Verification items for the finished model (mm, model axes). A direction names the side the tool comes from. Coordinates: 2 decimals unless noted, no trailing zeros. Write each loop counter-clockwise with the first axis right and the second up, starting at its lowest first coordinate (ties: lowest second). Pieces come first, ordered by that corner, then holes. Notation, with made-up numbers: (9.25, 45.5) -> (31.25, 45.5) arc R17 cw to (31.25, 50.5) -> close; hole circle Ø11 at (55.5, 83). An arc over 180 degrees is marked (long way). Answer in a Markdown table with one row per item.
Autodesk Inventor part; units mm, degrees
ref_plane "Work Plane1" through (0, 12, 0) normal (0, 1, 0) x (1, 0, 0)
ref_plane "YZ Plane" through (0, 0, 0) normal (1, 0, 0) x (0, 1, 0)
ref_plane "XZ Plane" through (0, 0, 0) normal (0, 1, 0) x (-1, 0, 0)
sketch "Sketch1" plane through (0, 0, 0) normal (0, 1, 0) x (-1, 0, 0)
  line L0 (0, 8.6603) -> (7.5, 4.3301)
  line L1 (7.5, 4.3301) -> (7.5, -4.3301)
  line L2 (7.5, -4.3301) -> (0, -8.6603)
  line L3 (0, -8.6603) -> (-7.5, -4.3301)
  line L4 (-7.5, -4.3301) -> (-7.5, 4.3301)
  line L5 (-7.5, 4.3301) -> (0, 8.6603)
  point P0 (0, 0)
  point P1 (0, 0)
  dimension "d0" = 7.5
extrude "Extrusion1" add sketch "Sketch1" along normal blind 6
ref_plane "Work Plane1" through (0, 12, 0) normal (0, 1, 0) x (1, 0, 0)
sketch "Sketch3" plane through (0, 12, 0) normal (0, 1, 0) x (1, 0, 0)
  circle A0 centre (0, 0) radius 0.75
  dimension "d4" = 1.5
loft "Loft1" add profiles "Sketch3" section 1 edges at (-3.75, 6, 6.4952) (3.75, 6, 6.4952) (7.5, 6, 0) (3.75, 6, -6.4952) (-3.75, 6, -6.4952) (-7.5, 6, 0)
sketch "Sketch4" plane through (0, 0, 0) normal (0, -1, 0) x (1, 0, 0)
  circle A0 centre (0, 0) radius 5
  dimension "d9" = 10
extrude "Extrusion2" cut sketch "Sketch4" against normal blind 6
thread "Thread1"
sketch "Sketch5" plane through (0, 6, 0) normal (0, -1, 0) x (1, 0, 0)
  circle A0 centre (0, 0) radius 5
  circle A1 centre (0, 0) radius 1.5875
  dimension "d14" = 3.175
sketch "Sketch6" plane through (0, 12, 0) normal (0, 1, 0) x (1, 0, 0)
  arc A0 (-0.6495, 0.375) -> (-0.6495, -0.375) centre (0, 0) ccw
  circle A1 centre (0, 0) radius 0.175
  dimension "d15" = 0.35
extrude "Extrusion3" cut sketch "Sketch6" against normal blind 7.75
extrude "Extrusion4" cut sketch "Sketch5" against normal blind 3.9 contours A1
chamfer "Chamfer1" distance 1.4 angle 45 1 edges at (-0.175, 9.9, 0)
properties part number "Nozzle"
1. Tool access check on faces 5 (the cylindrical face through (-0.34, 7.92, -1.55)), 6 (the flat face through (7.5, 3, 0)). Record the directions out of +Z, -Z, +X, -X, +Y, -Y that give a thin tool (end or side, any length) a straight path to the whole face; none if there is none.
Geometry says:
| item | result |
|---|---|
| face 5 | -Y |
| face 6 | +Z, -Z, +X, +Y, -Y |
2. Section check A-A, the plane y = 2.25. Record the boundary of the cut face in (x, z).
Geometry says:
| item | result |
|---|---|
| outline | (-7.5, -4.33) -> (0, -8.66) -> (7.5, -4.33) -> (7.5, 4.33) -> (0, 8.66) -> (-7.5, 4.33) -> close; hole circle Ø10 at (0, 0) |
3. Thickness scan on line 1 (X direction, y = 4, z = -4.5); line 2 (Z direction, x = -0.75, y = 5); line 3 (X direction, y = 2.25, z = -3). Record the ranges inside material, lowest first. Write a range as from..to.
Geometry says:
| item | result |
|---|---|
| line 1 | -7.21..-2.18, 2.18..7.21 |
| line 2 | -8.23..-4.94, 4.94..8.23 |
| line 3 | -7.5..-4, 4..7.5 |
4. Depth check by flat-ended pin: P1, Ø3, axis at x = 2.5, z = -2, coming from the -Y side; P2, Ø1.5, axis at x = 3, z = -4.5, coming from the +Y side; P3, Ø2.5, axis at x = 0, z = 0, coming from the +Y side; P4, Ø1.5, axis at x = 5.5, y = 3.5, coming from the -Z side. Enter the tip coordinate at first touch or a pass-through.
Geometry says:
| item | result |
|---|---|
| P1 | y = 6 |
| P2 | y = 8.54 |
| P3 | y = 12 |
| P4 | z = -5.92 |
5. Mould release check, pull along X, two halves, no side actions. Record for faces 1 (the flat face through (3.698, 2.958, -6.526)), 2 (the cylindrical face through (-1.08, 2.96, -4.88)), 3 (the flat face through (-3.698, 2.958, 6.526)), 4 (the flat face through (2, 6, 0)): released by +X, released by -X, zero draft, split by the parting line, or undercut.
Geometry says:
| item | result |
|---|---|
| face 1 | released by +X |
| face 2 | undercut |
| face 3 | released by -X |
| face 4 | undercut |
